```python
from build123d import *

# Parameters (mm, degrees)
SKETCH1_R           = 1.5
SKETCH1_R_2         = 95
BOSS_EXTRUDE1_DEPTH = 4.75


with BuildPart() as part:
    # Sketch1 → Boss-Extrude1 (new body)
    with BuildSketch(Plane.XY):
        with BuildLine():
            Line((-97.529258778, -78.185955787), (-60, -125))
            Line((-60, -125), (-60, -131))
            Line((-60, -131), (60, -131))
            Line((60, -131), (60, -125))
            Line((60, -125), (97.529258778, -78.185955787))
            ThreePointArc((97.529258778, -78.185955787), (0, 125), (-97.529258778, -78.185955787))
        make_face()
        with Locations((-77.781745931, -77.781745931)):
            Circle(SKETCH1_R, mode=Mode.SUBTRACT)
        with Locations((-20, -110)):
            Circle(SKETCH1_R, mode=Mode.SUBTRACT)
        with Locations((20, -110)):
            Circle(SKETCH1_R, mode=Mode.SUBTRACT)
        with Locations((77.781745931, -77.781745931)):
            Circle(SKETCH1_R, mode=Mode.SUBTRACT)
        with Locations((-110, 0)):
            Circle(SKETCH1_R, mode=Mode.SUBTRACT)
        with Locations((-77.781745931, 77.781745931)):
            Circle(SKETCH1_R, mode=Mode.SUBTRACT)
        Circle(SKETCH1_R_2, mode=Mode.SUBTRACT)
        with Locations((110, 0)):
            Circle(SKETCH1_R, mode=Mode.SUBTRACT)
        with Locations((0, 110)):
            Circle(SKETCH1_R, mode=Mode.SUBTRACT)
        with Locations((77.781745931, 77.781745931)):
            Circle(SKETCH1_R, mode=Mode.SUBTRACT)
    extrude(amount=BOSS_EXTRUDE1_DEPTH)


solid = part.part
```
Input: part model. Units: mm. Frame: model coordinates. Coordinates: 2 decimals unless noted, no trailing zeros. Write each loop counter-clockwise with the first axis right and the second up, starting at its lowest first coordinate (ties: lowest second). Pieces come first, ordered by that corner, then holes.
1) Material intervals for line 1 along Y through (x, z) = (-79, 1.05); line 2 along Y through (x, z) = (20, 1.3); line 3 along Y through (x, z) = (46, 3.5), sorted ascending.
2) Section C-C on z = 1.3. State how many separate pieces and enclosed holes the cut face has, and give its area (3 significant figures).
3) Pin query (flat end, axial travel): pin 1 Ø1.5 at (x, z) = (82, 2) entering from -Y; pin 2 Ø1.4 at (y, z) = (-127.5, 1.5) entering from +X; pin 3 Ø1.5 at (x, z) = (-40, 3) entering from +Y. Return the tip coordinate at first contact, or that it passes through.
4) Section A-A on y = -44. Output: boundary loops of the cut face in (x, z).
5) Section B-B on x = -88. Output: boundary loops of the cut face in (y, z) (3 decimals), and give its area (3 significant figures).
Check result:
1. line 1: y = -101.3 to -78.66, -76.91 to -52.76, 52.76 to 76.91, 78.66 to 96.87
1. line 2: y = -131 to -111.5, -108.5 to -92.87, 92.87 to 123.39
1. line 3: y = -131 to -83.12, 83.12 to 116.23
2. separate pieces: 1
2. enclosed holes: 10
2. area: 22,400 mm2
3. pin 1: stops at y = -98.49
3. pin 2: stops at x = 60
3. pin 3: stops at y = 118.68
4. outline: (-117, 0) - (-84.2, 0) - (-84.2, 4.75) - (-117, 4.75) - close; (84.2, 0) - (117, 0) - (117, 4.75) - (84.2, 4.75) - close
5. outline: (-90.073, 0) - (-35.791, 0) - (-35.791, 4.75) - (-90.073, 4.75) - close; (35.791, 0) - (88.775, 0) - (88.775, 4.75) - (35.791, 4.75) - close
5. area: 510 mm2
